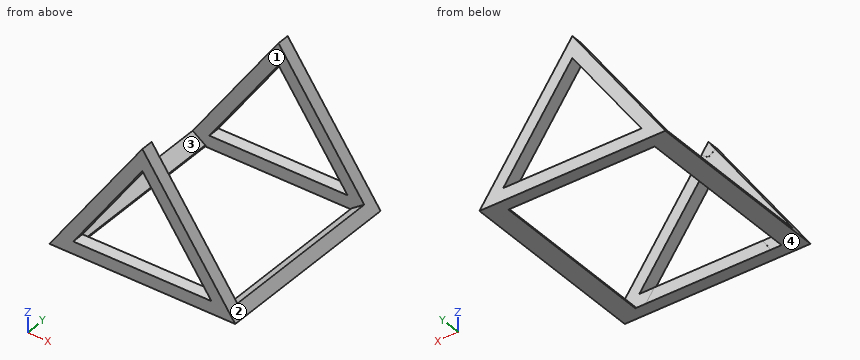
```python
from build123d import *

# Parameters (mm, degrees)
F1_DEPTH  = 400
F2_W      = 698.4
F2_H      = 562.6532291316
F3_DEPTH  = 101.6
F4_W      = 698.4
F4_H      = 562.6532291316
F5_DEPTH  = 101.6
F7_DEPTH  = 800.001
F8_W      = 599.9999940395
F8_H      = 698.1473760128
F9_DEPTH  = 584.2
F10_DEPTH = 101.6


with BuildPart() as f1:
    # F0 (on Front) → F1 (new body, symmetric)
    with BuildSketch(Plane.XZ):
        Polygon((0, 268.4965017427), (-381, -275.6278888261), (381, -275.6278888261), align=None)
    extrude(amount=F1_DEPTH, both=True)

    # F2 (on face) → F3 (cut)
    with BuildSketch(Plane(origin=(126.1520906972, 0, 88.3326448671), x_dir=(0, 1, 0), z_dir=(0.8191520443, 0, 0.5735764364))):
        with Locations((0, -112.1871562789)):
            Rectangle(F2_W, F2_H)
    extrude(amount=-F3_DEPTH, mode=Mode.SUBTRACT)

    # F4 (on face) → F5 (cut)
    with BuildSketch(Plane(origin=(-126.1520906972, 0, 88.3326448671), x_dir=(0, -1, 0), z_dir=(-0.8191520443, 0, 0.5735764364))):
        with Locations((0, -112.1871562789)):
            Rectangle(F4_W, F4_H)
    extrude(amount=-F5_DEPTH, mode=Mode.SUBTRACT)

    # F6 (on face) → F7 (cut, through all)
    with BuildSketch(Plane(origin=(0, 400, 0), x_dir=(-1, 0, 0), z_dir=(0, 1, 0))):
        Polygon((0, 179.9294045251), (-283.4141079499, -224.8278888261), (283.4141079499, -224.8278888261), align=None)
    extrude(amount=-F7_DEPTH, mode=Mode.SUBTRACT)

    # F8 (on face) → F9 (cut)
    with BuildSketch(Plane.XY.offset(-224.8278888261)):
        with Locations((-1.49012e-05, 0.1263119936)):
            Rectangle(F8_W, F8_H)
    extrude(amount=F9_DEPTH, mode=Mode.SUBTRACT)

    # F8 (on face) → F10 (cut)
    with BuildSketch(Plane.XY.offset(-224.8278888261)):
        with Locations((-1.49012e-05, 0.1263119936)):
            Rectangle(F8_W, F8_H)
    extrude(amount=-F10_DEPTH, mode=Mode.SUBTRACT)


solid = f1.part
```
Work out the finished part from the listing and answer in its coordinate system (mm). Face numbers are marked on the shaded views. Round coordinates to 2 decimals unless told otherwise and drop trailing zeros. Loops run counter-clockwise (first coordinate to the right, second up) from the corner with the lowest first, then second, coordinate; pieces in that order, holes last. Notation, with made-up numbers: M 59,86 L 102,86 A11 ccw 102,102 Z; hole C 16,51 d11. An arc over 180 degrees is marked long. One line per question, with ' | ' between items.
Q1. Find section D-D, the plane x = 326. Give the vertices of the cut face in (y, z).
Conclusion:
outline: M -400,-275.63 L 400,-275.63 L 400,-197.08 L 349.2,-197.08 L 349.2,-252.12 L -349.2,-252.12 L -349.2,-197.08 L -400,-197.08 Z
Q2. Each of these flat-tipped pins is pushed along its axis until it touches: pin 1 Ø4 at (y, z) = (-45, -273) entering from -X; pin 2 Ø6 at (y, z) = (-24.5, -272) entering from +X; pin 3 Ø15.5 at (x, y) = (74.5, -362) entering from +Z. Where does it stop, or does it pass through?
Conclusion:
pin 1: stops at x = -380.56 | pin 2: stops at x = 380.56 | pin 3: stops at z = 173.17
Q3. Consider line 1 along Y through (x, z) = (-26.5, 212.5); line 2 along Z through (x, y) = (79.5, 359.5); line 3 along Z through (x, y) = (320.5, -211.5). Determine where each line is inside the solid, lowest interval first. Write a range as from..to.
Conclusion:
line 1: y = -400..-349.2, 349.2..400 | line 2: z = -275.63..-224.83, 66.39..154.96 | line 3: z = -275.63..-255.98
Q4. Find section A-A, the plane y = -120. Give the vertices of the cut face in (x, z).
Conclusion:
outline: M -381,-275.63 L -300,-275.63 L -300,-270.33 L -351.86,-234.01 Z; M 300,-275.63 L 381,-275.63 L 351.86,-234.01 L 300,-270.33 Z
Q5. The mould has two halves that part along X. Classify the marked faces 1, 2, 3 and 4: +X half, -X half, draft (parallel to the pull), parting line (faces both ways), or undercut.
Conclusion:
face 1: undercut | face 2: +X half | face 3: undercut | face 4: draft
Q6. Find section C-C, the plane x = 173.5. Give the vertices of the cut face in (y, z), then the cut area to 3 significant figures.
Conclusion:
outline: M -400,-275.63 L -348.95,-275.63 L -348.95,-224.83 L -400,-224.83 Z; M -400,-67.85 L -349.2,-67.85 L -349.2,20.71 L -400,20.71 Z; M 349.2,-275.63 L 400,-275.63 L 400,-224.83 L 349.2,-224.83 Z; M 349.2,-67.85 L 400,-67.85 L 400,20.71 L 349.2,20.71 Z | area: 14,200 mm2
Q7. Find section B-B, the plane z = 70.5. Give the vertices of the cut face in (x, y).
Conclusion:
outline: M -138.64,-400 L -76.62,-400 L -76.62,-349.2 L -138.64,-349.2 Z; M -138.64,349.2 L -76.62,349.2 L -76.62,400 L -138.64,400 Z; M 76.62,-400 L 138.64,-400 L 138.64,-349.2 L 76.62,-349.2 Z; M 76.62,349.2 L 138.64,349.2 L 138.64,400 L 76.62,400 Z
